from build123d import *

# Parameters (mm, degrees)
SKETCH1_W               = 500
SKETCH1_H               = 300
BOSS_EXTRUDE1_DEPTH     = 1000
SKETCH2_W               = 440
SKETCH2_H               = 600
CUT_EXTRUDE1_DEPTH      = 1000
CUT_EXTRUDE1_DEPTH_BACK = 1000
SKETCH3_W               = 440
SKETCH3_H               = 330
CUT_EXTRUDE2_DEPTH      = 1000
CUT_EXTRUDE2_DEPTH_BACK = 1000
SKETCH4_W               = 240
SKETCH4_H               = 600
CUT_EXTRUDE3_DEPTH      = 1000
CUT_EXTRUDE3_DEPTH_BACK = 1000
SKETCH5_W               = 240
SKETCH5_H               = 330
CUT_EXTRUDE4_DEPTH      = 1000
CUT_EXTRUDE4_DEPTH_BACK = 1000


with BuildPart() as part:
    # Sketch1 → Boss-Extrude1 (new body)
    with BuildSketch(Plane(origin=(0, 0, 0), x_dir=(1, 0, 0), z_dir=(0, 1, 0))):
        Rectangle(SKETCH1_W, SKETCH1_H)
    extrude(amount=BOSS_EXTRUDE1_DEPTH)

    # Sketch2 → Cut-Extrude1 (cut, two sides)
    with BuildSketch(Plane.XY) as cut_extrude1_sk:
        with Locations((0, 660)):
            Rectangle(SKETCH2_W, SKETCH2_H)
    extrude(amount=CUT_EXTRUDE1_DEPTH, mode=Mode.SUBTRACT)
    extrude(cut_extrude1_sk.sketch, amount=-CUT_EXTRUDE1_DEPTH_BACK, mode=Mode.SUBTRACT)

    # Sketch3 → Cut-Extrude2 (cut, two sides)
    with BuildSketch(Plane.XY) as cut_extrude2_sk:
        with Locations((0, 165)):
            Rectangle(SKETCH3_W, SKETCH3_H)
    extrude(amount=CUT_EXTRUDE2_DEPTH, mode=Mode.SUBTRACT)
    extrude(cut_extrude2_sk.sketch, amount=-CUT_EXTRUDE2_DEPTH_BACK, mode=Mode.SUBTRACT)

    # Sketch4 → Cut-Extrude3 (cut, two sides)
    with BuildSketch(Plane(origin=(0, 0, 0), x_dir=(0, 0, -1), z_dir=(1, 0, 0))) as cut_extrude3_sk:
        with Locations((0, 660)):
            Rectangle(SKETCH4_W, SKETCH4_H)
    extrude(amount=CUT_EXTRUDE3_DEPTH, mode=Mode.SUBTRACT)
    extrude(cut_extrude3_sk.sketch, amount=-CUT_EXTRUDE3_DEPTH_BACK, mode=Mode.SUBTRACT)

    # Sketch5 → Cut-Extrude4 (cut, two sides)
    with BuildSketch(Plane(origin=(0, 0, 0), x_dir=(0, 0, -1), z_dir=(1, 0, 0))) as cut_extrude4_sk:
        with Locations((0, 165)):
            Rectangle(SKETCH5_W, SKETCH5_H)
    extrude(amount=CUT_EXTRUDE4_DEPTH, mode=Mode.SUBTRACT)
    extrude(cut_extrude4_sk.sketch, amount=-CUT_EXTRUDE4_DEPTH_BACK, mode=Mode.SUBTRACT)


solid = part.part
Could you check a few things on this model? Use its own coordinates, in mm. A direction names the side the tool comes from. Coordinates: 2 decimals unless noted, no trailing zeros. Order: outer loops, then holes, each group sorted by start corner. A loop starts at its lowest first (then second) coordinate and runs counter-clockwise, first axis right, second up. Notation, with made-up numbers: (-24, -15.5) -> (19, -15.5) arc R23 cw to (19, 21.5) -> close; hole circle Ø4 at (32.5, -10). An arc over 180 degrees is marked (long way). One line per item, written item: value. Start each with the question number.
1) If I drill on L1, parallel to Y at x = 135.5, z = -22; L2, parallel to X at y = 195, z = 124, over which ranges is the centre line in solid material (lowest first)? Write a range as [from, to].
2) Imagine slicing it at C-C on x = -196. List the corners of the cut face in (y, z) for me, plus the area to 3 significant figures.
3) We'd pull the mould along Z, two halves only. Please class faces 5 (the flat face through (-235, 656, -120)), 6 (the flat face through (-220, 656, -135)), 7 (the flat face through (-1, 350, -150)), 8 (the flat face through (-1, 350, 150)): +Z half, -Z half, draft (parallel to the pull), parting line (faces both ways), or undercut.
4) Imagine slicing it at A-A on y = 735. List the corners of the cut face in (x, z) for me.
5) Which directions (+Z, -Z, +X, -X, +Y, -Y) give clear straight access to the entire face, cutting with the end or side of a thin tool? Please do faces 1 (the flat face through (220, 163, -135)), 2 (the flat face through (235, 656, -120)), 3 (the flat face through (-220, 656, 135)), 4 (the flat face through (235, 163, 120)).
6) I'm going to push a flat-ended pin straight in: pin 1 (10 mm diameter, centred on x = 95, z = -117.5, fed in from -Y). Where does the tip first touch, or does it pass through?
7) Imagine slicing it at B-B on z = 32. List the corners of the cut face in (x, y) for me, plus the area to 3 significant figures.
Answer list:
1. L1: y = [330, 360], [960, 1000]
1. L2: x = [-250, -220], [220, 250]
2. outline: (330, -150) -> (360, -150) -> (360, 150) -> (330, 150) -> close; (960, -150) -> (1000, -150) -> (1000, 150) -> (960, 150) -> close
2. area: 21,000 mm2
3. face 5: undercut
3. face 6: draft
3. face 7: -Z half
3. face 8: +Z half
4. outline: (-250, -150) -> (-220, -150) -> (-220, -120) -> (-250, -120) -> close; (-250, 120) -> (-220, 120) -> (-220, 150) -> (-250, 150) -> close; (220, -150) -> (250, -150) -> (250, -120) -> (220, -120) -> close; (220, 120) -> (250, 120) -> (250, 150) -> (220, 150) -> close
5. face 1: +Z, -Z, -Y
5. face 2: +X, -X
5. face 3: +Z, -Z
5. face 4: +X, -X, -Y
6. pin 1: stops at y = 330
7. outline: (-250, 330) -> (250, 330) -> (250, 360) -> (-250, 360) -> close; (-250, 960) -> (250, 960) -> (250, 1000) -> (-250, 1000) -> close
7. area: 35,000 mm2
